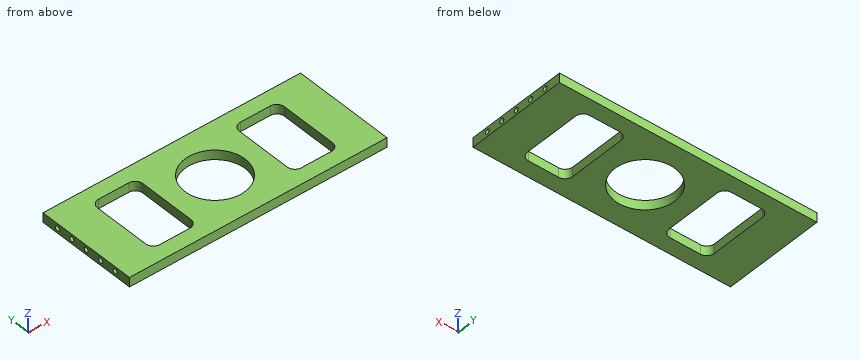
Autodesk Inventor part; units mm, degrees
ref_plane "YZ Plane" through (0, 0, 0) normal (1, 0, 0) x (0, 1, 0)
ref_plane "XZ Plane" through (0, 0, 0) normal (0, 1, 0) x (-1, 0, 0)
ref_plane "XY Plane" through (0, 0, 0) normal (0, 0, 1) x (1, 0, 0)
sketch "스케치1" plane through (0, 0, 0) normal (0, 0, 1) x (1, 0, 0)
  line L0 (-68.5, 27) -> (68.5, 27)
  line L1 (68.5, 27) -> (68.5, -27)
  line L2 (68.5, -27) -> (-68.5, -27)
  line L3 (-68.5, -27) -> (-68.5, 27)
  point P0 (0, 0)
  dimension "d0" = 137
  dimension "d1" = 54
  dimension "d2" = 27
  dimension "d3" = 68.5
extrude "돌출1" add sketch "스케치1" along normal blind 5
sketch "스케치2" plane through (-68.5, -27, 0) normal (-1, 0, 0) x (0, 0, 1)
  line L0 (0, 54) -> (0, 0)
  line L1 (0, 0) -> (5, 0)
  line L2 (5, 0) -> (51, 4)
  line L3 (51, 50) -> (5, 54)
  line L4 (5, 54) -> (0, 54)
  circle A0 centre (2.5, 9) radius 1.25
  circle A1 centre (2.5, 18) radius 1.25
  circle A2 centre (2.5, 27) radius 1.25
  circle A3 centre (2.5, 36) radius 1.25
  circle A4 centre (2.5, 45) radius 1.25
  line L5 (0, 0) -> (0, 54)
  line L6 (0, 0) -> (5, 0)
  line L7 (5, 54) -> (5, 0)
  line L8 (0, 54) -> (5, 54)
  point P0 (0, 27)
  dimension "d6" = 2.5
  dimension "d7" = 2.5
  dimension "d8" = 2.5
  dimension "d9" = 2.5
  dimension "d10" = 2.5
  dimension "d11" = 2.5
  dimension "d12" = 2.5
  dimension "d13" = 2.5
  dimension "d14" = 2.5
  dimension "d15" = 2.5
  dimension "d16" = 9
  dimension "d17" = 18
  dimension "d18" = 27
  dimension "d19" = 36
  dimension "d20" = 9
extrude "돌출2" cut sketch "스케치2" against normal blind 10 contours A0 | A1 | A2 | A3 | A4
sketch "스케치3" plane through (68.5, -27, 0) normal (1, 0, 0) x (0, 0, -1)
  line L0 (0, 0) -> (0, 54)
  line L1 (0, 54) -> (-5, 54)
  line L2 (-5, 54) -> (-51, 50)
  line L3 (-51, 4) -> (-5, 0)
  line L4 (-5, 0) -> (0, 0)
  circle A0 centre (-2.5, 45) radius 1.25
  circle A1 centre (-2.5, 36) radius 1.25
  circle A2 centre (-2.5, 27) radius 1.25
  circle A3 centre (-2.5, 18) radius 1.25
  circle A4 centre (-2.5, 9) radius 1.25
  line L5 (0, 54) -> (0, 0)
  line L6 (0, 54) -> (-5, 54)
  line L7 (-5, 0) -> (-5, 54)
  line L8 (0, 0) -> (-5, 0)
  point P0 (0, 27)
  dimension "d23" = 2.5
  dimension "d24" = 2.5
  dimension "d25" = 2.5
  dimension "d26" = 2.5
  dimension "d27" = 2.5
  dimension "d28" = 2.5
  dimension "d29" = 2.5
  dimension "d30" = 2.5
  dimension "d31" = 2.5
  dimension "d32" = 2.5
  dimension "d33" = 9
  dimension "d34" = 18
  dimension "d35" = 27
  dimension "d36" = 36
  dimension "d37" = 9
extrude "돌출3" cut sketch "스케치3" against normal blind 10 contours A0 | A1 | A2 | A3 | A4
sketch "스케치5" plane through (0, 0, 5) normal (0, 0, 1) x (1, 0, 0)
  line L0 (68.5, 27) -> (-68.5, 27)
  line L1 (-68.5, 27) -> (-68.5, -27)
  line L2 (-68.5, -27) -> (68.5, -27)
  line L3 (68.5, -27) -> (68.5, 27)
  line L4 (68.5, 27) -> (-68.5, 27)
  line L5 (-68.5, -0.0341) -> (68.5, 0) construction
  line L6 (-45.6619, 19) -> (-29.6619, 19)
  line L7 (-25.6619, 15) -> (-25.6619, -15.0528)
  line L8 (-29.6619, -19.0528) -> (-45.6619, -19.0528)
  line L9 (-49.6619, -15.0528) -> (-49.6619, 15)
  line L10 (-49.6619, 19) -> (-25.6619, -19.0528) construction
  line L11 (-25.6619, 19) -> (-49.6619, -19.0528) construction
  arc A0 (-45.6619, 19) -> (-49.6619, 15) centre (-45.6619, 15) ccw
  arc A1 (-25.6619, 15) -> (-29.6619, 19) centre (-29.6619, 15) ccw
  arc A2 (-29.6619, -19.0528) -> (-25.6619, -15.0528) centre (-29.6619, -15.0528) ccw
  arc A3 (-49.6619, -15.0528) -> (-45.6619, -19.0528) centre (-45.6619, -15.0528) ccw
  line L12 (0, 29) -> (0, -29)
  arc A4 (29.6619, 19) -> (25.6619, 15) centre (29.6619, 15) ccw
  line L13 (25.6619, 15) -> (25.6619, -15.0528)
  arc A5 (25.6619, -15.0528) -> (29.6619, -19.0528) centre (29.6619, -15.0528) ccw
  line L14 (45.6619, 19) -> (29.6619, 19)
  arc A6 (49.6619, 15) -> (45.6619, 19) centre (45.6619, 15) ccw
  line L15 (49.6619, 19) -> (25.6619, -19.0528) construction
  line L16 (25.6619, 19) -> (49.6619, -19.0528) construction
  line L17 (49.6619, -15.0528) -> (49.6619, 15)
  arc A7 (45.6619, -19.0528) -> (49.6619, -15.0528) centre (45.6619, -15.0528) ccw
  line L18 (29.6619, -19.0528) -> (45.6619, -19.0528)
  point P0 (0, 0)
  point P1 (-37.6619, -0.0264)
  point P2 (37.6619, -0.0264)
  point P3 (0, 0)
  dimension "d85" = 24
  dimension "d86" = 4
extrude "돌출4" cut sketch "스케치5" against normal up to surface (5 mm away) contours L6 A1 L7 A2 L8 A3 L9 A0 | L14 A6 L17 A7 L18 A5 L13 A4
sketch "스케치9" plane through (0, 0, 5) normal (0, 0, 1) x (1, 0, 0)
  circle A0 centre (0, 0) radius 16
  dimension "d82" = 32
extrude "돌출8" cut sketch "스케치9" against normal blind 10
properties part number "J2L1_H_Top" material "알루미늄 6061"
The model under review builds one solid part; all positions refer to its coordinate system, in mm. Coordinates: 2 decimals unless noted, no trailing zeros. Write each loop counter-clockwise with the first axis right and the second up, starting at its lowest first coordinate (ties: lowest second). Pieces come first, ordered by that corner, then holes. Notation, with made-up numbers: (24.5, -12.75) - (68.5, -12.75) arc R22 cw to (68.5, 0.25) - close; hole circle Ø7 at (0.5, -34). An arc over 180 degrees is marked (long way). Answer as a JSON object with one key per item and string values. Group by question number.
1. Add section D-D (x = 0). Give the boundary of the cut face in (y, z).
2. Clearance check with flat-ended pins moving along their axes: pin 1 Ø1 at (y, z) = (10, 2.5) entering from -X; pin 2 Ø0.8 at (y, z) = (9.5, 2.5) entering from +X; pin 3 Ø2 at (y, z) = (-9, 2.5) entering from -X. State where each tip first meets the part, or that it passes through.
3. To check wall thickness, follow probe 1 along Y at (x, z) = (64.75, 2.5); probe 2 along Y at (x, z) = (41, 2.7); probe 3 along X at (y, z) = (-6, 2.1). State the ranges of each line that lie inside material, in increasing order.
4. Add section B-B (x = 39). Give the boundary of the cut face in (y, z).
5. Add section C-C (z = 2.5). Give the number of separate pieces and of enclosed holes in the cut face, plus the area to 3 significant figures.
6. Add section A-A (y = 0). Give the boundary of the cut face in (x, z), plus the area to 3 significant figures.
Findings:
{
 "1": {"outline": "(-27, 0) - (-16, 0) - (-16, 5) - (-27, 5) - close; (16, 0) - (27, 0) - (27, 5) - (16, 5) - close"},
 "2": {"pin 1": "x = -68.5", "pin 2": "x = 58.5", "pin 3": "x = -58.5"},
 "3": {"probe 1": "-27 to -19.25, -16.75 to -10.25, -7.75 to -1.25, 1.25 to 7.75, 10.25 to 16.75, 19.25 to 27", "probe 2": "-27 to -19.05, 19 to 27", "probe 3": "-68.5 to -49.66, -25.66 to -14.83, 14.83 to 25.66, 49.66 to 68.5"},
 "4": {"outline": "(-27, 0) - (-19.05, 0) - (-19.05, 5) - (-27, 5) - close; (19, 0) - (27, 0) - (27, 5) - (19, 5) - close"},
 "5": {"separate pieces": "1", "enclosed holes": "3", "area": "4,540 mm²"},
 "6": {"outline": "(-68.5, 0) - (-49.66, 0) - (-49.66, 5) - (-68.5, 5) - (-68.5, 3.75) - (-58.5, 3.75) - (-58.5, 1.25) - (-68.5, 1.25) - close; (-25.66, 0) - (-16, 0) - (-16, 5) - (-25.66, 5) - close; (16, 0) - (25.66, 0) - (25.66, 5) - (16, 5) - close; (49.66, 0) - (68.5, 0) - (68.5, 1.25) - (58.5, 1.25) - (58.5, 3.75) - (68.5, 3.75) - (68.5, 5) - (49.66, 5) - close", "area": "235 mm²"}
}
